Geometry: final body of the model. Coordinates: model frame, mm. Face numbers are marked on the shaded views. A direction names the side the tool comes from. Give positions to 0.01 mm unless a question says otherwise; leave off trailing zeros. Order: outer loops, then holes, each group sorted by start corner. A loop starts at its lowest first (then second) coordinate and runs counter-clockwise, first axis right, second up. Notation, with made-up numbers: (76.25, 37) - (130.25, 37) arc R18 ccw to (130.25, 54) - close; hole circle Ø4 at (-31.75, 86). An arc over 180 degrees is marked (long way). One line per item, written item: value.
```python
from build123d import *

# Parameters (mm, degrees)
SKETCH1_W           = 39
SKETCH1_H           = 34.4
SKETCH1_R           = 1.6
BOSS_EXTRUDE5_DEPTH = 4
FILLET1_R           = 5
BOSS_EXTRUDE6_START = -2.6
SKETCH4_R           = 2.6
SKETCH4_R_2         = 1.6
BOSS_EXTRUDE6_DEPTH = 2.6
FILLET4_R           = 2
FILLET5_R           = 2
FILLET6_R           = 2
FILLET8_R           = 2
FILLET9_R           = 2
FILLET10_R          = 2
FILLET11_R          = 2
FILLET12_R          = 2
FILLET13_R          = 2
FILLET14_R          = 2
FILLET15_R          = 2
FILLET16_R          = 2


with BuildPart() as part:
    # Sketch1 → Boss-Extrude5 (new body)
    with BuildSketch(Plane.XY):
        with Locations((0.200050248, -2.49430892)):
            Rectangle(SKETCH1_W, SKETCH1_H)
        with Locations((-14.999949752, 9.50569108)):
            Circle(SKETCH1_R, mode=Mode.SUBTRACT)
        with Locations((15.400050248, 9.50569108)):
            Circle(SKETCH1_R, mode=Mode.SUBTRACT)
        with Locations((-14.999949752, -14.49430892)):
            Circle(SKETCH1_R, mode=Mode.SUBTRACT)
        with Locations((15.400050248, -14.49430892)):
            Circle(SKETCH1_R, mode=Mode.SUBTRACT)
        Polygon((14.300050248, 0.15569108), (11.300050248, 0.15569108), (11.300050248, 8.00569108), (-10.899949752, 8.00569108), (-10.899949752, 0.15569108), (-13.899949752, 0.15569108), (-13.899949752, -5.14430892), (-10.899949752, -5.14430892), (-10.899949752, -12.99430892), (11.300050248, -12.99430892), (11.300050248, -5.14430892), (14.300050248, -5.14430892), align=None, mode=Mode.SUBTRACT)
    extrude(amount=BOSS_EXTRUDE5_DEPTH)

    # Fillet1
    fillet1_edges = [part.edges().sort_by_distance(p)[0] for p in [
        (-19.299949752, 14.70569108, 2),
        (19.700050248, 14.70569108, 2),
    ]]
    fillet(fillet1_edges, radius=FILLET1_R)

    # Sketch4 → Boss-Extrude6 (add)
    # profile 1 of 4: a face of its own
    with BuildSketch(Plane.XY.offset(BOSS_EXTRUDE6_START)):
        with Locations((15.400050248, 9.50569108)):
            Circle(SKETCH4_R)
        with Locations((15.400050248, 9.50569108)):
            Circle(SKETCH4_R_2, mode=Mode.SUBTRACT)
    # profile 2 of 4: a face of its own
    with BuildSketch(Plane.XY.offset(BOSS_EXTRUDE6_START)):
        with Locations((-14.999949752, 9.50569108)):
            Circle(SKETCH4_R)
        with Locations((-14.999949752, 9.50569108)):
            Circle(SKETCH4_R_2, mode=Mode.SUBTRACT)
    # profile 3 of 4: a face of its own
    with BuildSketch(Plane.XY.offset(BOSS_EXTRUDE6_START)):
        with Locations((15.400050248, -14.49430892)):
            Circle(SKETCH4_R)
        with Locations((15.400050248, -14.49430892)):
            Circle(SKETCH4_R_2, mode=Mode.SUBTRACT)
    # profile 4 of 4: a face of its own
    with BuildSketch(Plane.XY.offset(BOSS_EXTRUDE6_START)):
        with Locations((-14.999949752, -14.49430892)):
            Circle(SKETCH4_R)
        with Locations((-14.999949752, -14.49430892)):
            Circle(SKETCH4_R_2, mode=Mode.SUBTRACT)
    extrude(amount=BOSS_EXTRUDE6_DEPTH)

    # Fillet4
    fillet4_edges = [part.edges().sort_by_distance(p)[0] for p in [
        (-10.899949752, 8.00569108, 2),
    ]]
    fillet(fillet4_edges, radius=FILLET4_R)

    # Fillet5
    fillet5_edges = [part.edges().sort_by_distance(p)[0] for p in [
        (-10.899949752, 0.15569108, 2),
    ]]
    fillet(fillet5_edges, radius=FILLET5_R)

    # Fillet6
    fillet6_edges = [part.edges().sort_by_distance(p)[0] for p in [
        (-13.899949752, 0.15569108, 2),
    ]]
    fillet(fillet6_edges, radius=FILLET6_R)

    # Fillet8
    fillet8_edges = [part.edges().sort_by_distance(p)[0] for p in [
        (-13.899949752, -5.14430892, 2),
    ]]
    fillet(fillet8_edges, radius=FILLET8_R)

    # Fillet9
    fillet9_edges = [part.edges().sort_by_distance(p)[0] for p in [
        (-10.899949752, -5.14430892, 2),
    ]]
    fillet(fillet9_edges, radius=FILLET9_R)

    # Fillet10
    fillet10_edges = [part.edges().sort_by_distance(p)[0] for p in [
        (-10.899949752, -12.99430892, 2),
    ]]
    fillet(fillet10_edges, radius=FILLET10_R)

    # Fillet11
    fillet11_edges = [part.edges().sort_by_distance(p)[0] for p in [
        (11.300050248, -5.14430892, 2),
    ]]
    fillet(fillet11_edges, radius=FILLET11_R)

    # Fillet12
    fillet12_edges = [part.edges().sort_by_distance(p)[0] for p in [
        (11.300050248, 0.15569108, 2),
    ]]
    fillet(fillet12_edges, radius=FILLET12_R)

    # Fillet13
    fillet13_edges = [part.edges().sort_by_distance(p)[0] for p in [
        (11.300050248, -12.99430892, 2),
    ]]
    fillet(fillet13_edges, radius=FILLET13_R)

    # Fillet14
    fillet14_edges = [part.edges().sort_by_distance(p)[0] for p in [
        (14.300050248, 0.15569108, 2),
    ]]
    fillet(fillet14_edges, radius=FILLET14_R)

    # Fillet15
    fillet15_edges = [part.edges().sort_by_distance(p)[0] for p in [
        (11.300050248, 8.00569108, 2),
    ]]
    fillet(fillet15_edges, radius=FILLET15_R)

    # Fillet16
    fillet16_edges = [part.edges().sort_by_distance(p)[0] for p in [
        (14.300050248, -5.14430892, 2),
    ]]
    fillet(fillet16_edges, radius=FILLET16_R)


solid = part.part
```
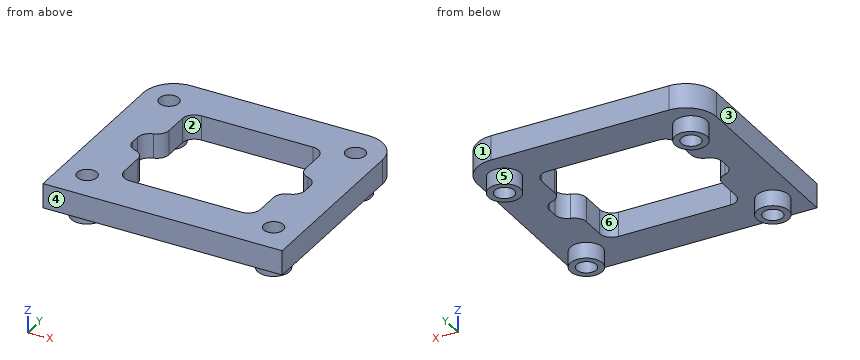
1) Section C-C, the plane x = 16.5. Return loops of the section in (y, z).
Answers below:
outline: (-19.69, 0) - (-16.85, 0) - (-16.85, -2.6) - (-15.66, -2.6) - (-15.66, 4) - (-19.69, 4) - close; (-13.33, -2.6) - (-12.14, -2.6) - (-12.14, 0) - (7.15, 0) - (7.15, -2.6) - (8.34, -2.6) - (8.34, 4) - (-13.33, 4) - close; (10.67, -2.6) - (11.86, -2.6) - (11.86, 0) - (14.37, 0) - (14.37, 4) - (10.67, 4) - close
2) Section D-D, the plane x = 10.5. Return loops of the section in (y, z), then the cut area to 3 significant figures.
Answers below:
outline: (-19.69, 0) - (-12.59, 0) - (-12.59, 4) - (-19.69, 4) - close; (7.61, 0) - (14.71, 0) - (14.71, 4) - (7.61, 4) - close
area: 56.8 mm^2
3) Section B-B, the plane z = -1. Return loops of the section in (x, y).
Answers below:
outline: circle Ø5.2 at (-15, -14.49); circle Ø5.2 at (-15, 9.51); circle Ø5.2 at (15.4, -14.49); circle Ø5.2 at (15.4, 9.51); hole circle Ø3.2 at (-15, -14.49); hole circle Ø3.2 at (-15, 9.51); hole circle Ø3.2 at (15.4, -14.49); hole circle Ø3.2 at (15.4, 9.51)
4) Material intervals for line 1 along Y through (x, z) = (-8, 0.25); line 2 along X through (y, z) = (9, 2.25); line 3 along X through (y, z) = (-15.5, 2.25), sorted ascending.
Answers below:
line 1: -19.69 to -12.99, 8.01 to 14.71
line 2: -19.3 to -16.52, -13.48 to 13.88, 16.92 to 19.7
line 3: -19.3 to -16.24, -13.76 to 14.16, 16.64 to 19.7
5) Mould query, pull axis Y, two halves, no side actions, for the marked faces 1, 2 and 3. Classes: released by +Y, released by -Y, zero draft, split by the parting line, or undercut.
Answers below:
face 1: released by +Y
face 2: undercut
face 3: zero draft
6) Set-up query: the marked faces 4, 5 and 6. Return all of +Z, -Z, +X, -X, +Y, -Y with unobstructed straight access to the full face (end or side cutting, diameter ignored); none if empty.
Answers below:
face 4: +Z, -Z, +X, -X, -Y
face 5: -Z
face 6: +Z, -Z
7) First-contact query: pin 1 (4 mm diameter, centred on x = 15.4, y = -14.49, fed in from +Z); pin 2 (3 mm diameter, centred on x = -10.5, y = -0.5, fed in from -Z); pin 3 (17 mm diameter, centred on x = 7, y = -6.5, fed in from -Z). Flat tips, straight axial feed; report the tip coordinate or a pass-through.
Answers below:
pin 1: z = 4
pin 2: through
pin 3: z = 0
8) Section A-A, the plane y = 4. Return loops of the section in (x, z), then the cut area to 3 significant figures.
Answers below:
outline: (-19.3, 0) - (-10.9, 0) - (-10.9, 4) - (-19.3, 4) - close; (11.3, 0) - (19.7, 0) - (19.7, 4) - (11.3, 4) - close
area: 67.2 mm^2
